The listing builds one solid part. Answer for the finished solid, in the listing's coordinates (mm). Face numbers are marked on the shaded views. A direction names the side the tool comes from. Give positions to 0.01 mm unless a question says otherwise; leave off trailing zeros. Order: outer loops, then holes, each group sorted by start corner. A loop starts at its lowest first (then second) coordinate and runs counter-clockwise, first axis right, second up. Notation, with made-up numbers: (-9, -17.5) - (3, -17.5) arc R6 ccw to (3, -11.5) - close; hole circle Ø11 at (56.5, 2.25). An arc over 180 degrees is marked (long way). Answer as a JSON object with one key per item and string values. Group by question number.
Q1. For the marked faces 1 and 2, determine the directions among +Z, -Z, +X, -X, +Y, -Y from which every point of the face is accessible in a straight line to the end or side of a thin tool.
Q2. Given pin 1 (3 mm diameter, centred on y = -14, z = 0, fed in from +X), flat-ended and moving along its own axis, determine where the tip first touches the part or whether it passes through.
Q3. Consider line 1 (Y direction, x = 0.3, z = 0); line 2 (Z direction, x = -0.8, y = -14); line 3 (Y direction, x = -0.5, z = -0.5). Determine where each line is inside the solid, lowest interval first.
Q4. A cutting plane is placed at B-B, the plane y = -14. Give the vertices of the cut face in (x, z), and give its area (3 significant figures).
Q5. The mould has two halves that part along Y. Classify the marked faces 3 and 4: released by +Y, released by -Y, zero draft, split by the parting line, or undercut.
Q6. A cutting plane is placed at A-A, the plane z = 0. Give the vertices of the cut face in (x, y), and give its area (3 significant figures).
Q7. A cutting plane is placed at C-C, the plane y = 0. Give the vertices of the cut face in (x, z), and give its area (4 significant figures).
Autodesk Inventor part; units mm, degrees
ref_plane "YZ Plane" through (0, 0, 0) normal (1, 0, 0) x (0, 1, 0)
ref_plane "XZ Plane" through (0, 0, 0) normal (0, 1, 0) x (-1, 0, 0)
ref_plane "XY Plane" through (0, 0, 0) normal (0, 0, 1) x (1, 0, 0)
sketch "Sketch1" plane through (0, 0, 0) normal (1, 0, 0) x (0, 1, 0)
  circle A0 centre (-14, 0) radius 3
  circle A1 centre (14, 0) radius 3
  line L0 (-14, 0) -> (14, 0) construction
  point P0 (0, 0)
  point P1 (0, 0)
  dimension "d0" = 6
  dimension "d1" = 28
extrude "Extrusion1" add sketch "Sketch1" along normal mid plane 3
sketch "Sketch2" plane through (1.5, 14, 0) normal (1, 0, 0) x (0, 0, -1)
  circle A0 centre (0, -28) radius 3
  circle A1 centre (0, 0) radius 3
  circle A2 centre (0, -28) radius 3
  arc A3 (-2.9319, -27.3644) -> (-2.9319, -0.6356) centre (-64.5833, -14) ccw
  arc A4 (2.9319, -0.6356) -> (2.9319, -27.3644) centre (64.5833, -14) ccw
  circle A5 centre (0, 0) radius 3
  point P0 (0, -14)
  dimension "d4" = 3
extrude "Extrusion2" add sketch "Sketch2" against normal blind 1.5 contours A0 A3 A1 A4
sketch "Sketch3" plane through (1.5, 0, 0) normal (1, 0, 0) x (0, 0, -1)
  arc A0 (-2.9319, -13.3644) -> (2.9319, -13.3644) centre (0, -14) ccw
  arc A1 (2.9319, 13.3644) -> (2.9319, -13.3644) centre (64.5833, 0) ccw
  arc A2 (2.9319, 13.3644) -> (-2.9319, 13.3644) centre (0, 14) ccw
  arc A3 (-2.9319, -13.3644) -> (-2.9319, 13.3644) centre (-64.5833, 0) ccw
  point P0 (0, 0)
hole "Hole1" at (1.5, 14, 0) at (1.5, -14, 0) direction (-1, 0, 0) diameter 2.459 end through all
chamfer "Chamfer1" distance 0.25 angle 45 9 edges at (1.5, 0, 1.5) (1.5, -17, 0) (1.5, 0, -1.5) (1.5, 15.8833, -2.3352) (1.5, 15.8833, 2.3352) (-1.5, 11, 0) (-1.5, -17, 0) (0, 0, -1.5) (0, 0, 1.5)
properties part number "Backplane_CenterNut" material "Aluminum"
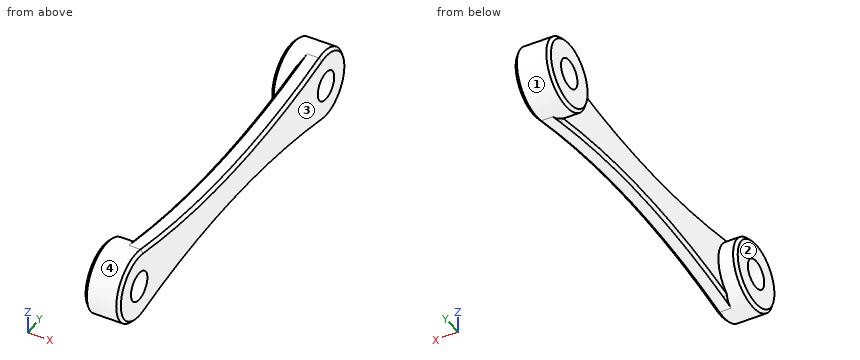
Reply:
{
 "1": {"face 1": "-X", "face 2": "+Z, -Z, -X, +Y, -Y"},
 "2": {"pin 1": "stops at x = 1.5"},
 "3": {"line 1": "y = -17 to -15.23, -12.77 to 12.77, 15.23 to 17", "line 2": "z = -3 to -1.23, 1.23 to 3", "line 3": "y = -16.96 to -15.12, -12.88 to -11.04, 11.04 to 12.88, 15.12 to 16.96"},
 "4": {"outline": "(-1.5, -2.75) - (-1.25, -3) - (1.25, -3) - (1.5, -2.75) - (1.5, -1.23) - (-1.5, -1.23) - close; (-1.5, 1.23) - (1.5, 1.23) - (1.5, 2.75) - (1.25, 3) - (-1.25, 3) - (-1.5, 2.75) - close", "area": "10.5 mm^2"},
 "5": {"face 3": "zero draft", "face 4": "undercut"},
 "6": {"outline": "(-1.5, -16.75) - (-1.25, -17) - (1.25, -17) - (1.5, -16.75) - (1.5, -15.23) - (-1.5, -15.23) - close; (-1.5, -12.77) - (1.5, -12.77) - (1.5, 12.77) - (-1.5, 12.77) - (-1.5, 11.25) - (-1.25, 11) - (0, 11) - (0, -11) - (-1.25, -11) - (-1.5, -11.25) - close; (-1.5, 15.23) - (1.5, 15.23) - (1.5, 16.75) - (1.25, 17) - (-1.25, 17) - (-1.5, 16.75) - close", "area": "54.1 mm^2"},
 "7": {"outline": "(0, -1.25) - (0.25, -1.5) - (1.25, -1.5) - (1.5, -1.25) - (1.5, 1.25) - (1.25, 1.5) - (0.25, 1.5) - (0, 1.25) - close", "area": "4.375 mm^2"}
}
